```python
from build123d import *

# Parameters (mm, degrees)
SKETCH1_W                = 11
SKETCH1_H                = 10.5
BOSS_EXTRUDE1_DEPTH      = 7.5
SKETCH2_W                = 11
SKETCH2_H                = 10.5
SKETCH2_R                = 2.795278083
CUT_EXTRUDE1_DEPTH       = 6
CUT_EXTRUDE2_DEPTH       = 6
SKETCH5_W                = 5.867744682
SKETCH5_H                = 6.773951876
SKETCH5_W_2              = 3.131118199
SKETCH5_H_2              = 7.595162723
SKETCH5_W_3              = 1.565559099
SKETCH5_H_3              = 1.410160094
SKETCH5_W_4              = 1.497318165
SKETCH5_W_5              = 1.429294678
SKETCH5_W_6              = 1.22939712
BOSS_EXTRUDE2_DEPTH      = 0.5
SKETCH6_R                = 0.720165483
CUT_EXTRUDE3_DEPTH       = 5.5
CUT_EXTRUDE4_START       = -0.5
SKETCH7_W                = 6.315969547
SKETCH7_H                = 7.313839146
SKETCH7_R                = 1.792834501
CUT_EXTRUDE4_DEPTH       = 4.5
SKETCH8_W                = 2.504754688
SKETCH8_H                = 5.654171149
BOSS_EXTRUDE3_DEPTH      = 2.5
CHAMFER1_SIZE            = 0.5
BOSS_EXTRUDE4_DEPTH      = 0.5
BOSS_EXTRUDE4_DEPTH_BACK = 6
SKETCH11_R               = 0.448273795
SKETCH11_R_2             = 0.519161878
SKETCH11_R_3             = 0.470017501
SKETCH11_R_4             = 0.405329815
CUT_EXTRUDE5_DEPTH       = 6
SKETCH12_W               = 15.986280265
SKETCH12_H               = 22.221265256
CUT_EXTRUDE6_DEPTH       = 1
SKETCH14_W               = 2.367247422
SKETCH14_H               = 5.32267157
SKETCH14_W_2             = 2.25297781
SKETCH14_W_3             = 3.874113275
SKETCH14_H_2             = 2.566072862
BOSS_EXTRUDE5_DEPTH      = 1
SKETCH15_W               = 0.295662385
SKETCH15_H               = 1.277257847
SKETCH15_W_2             = 2.29913968
SKETCH15_H_2             = 1.589846546
BOSS_EXTRUDE6_DEPTH      = 0.25


with BuildPart() as part:
    # Sketch1 → Boss-Extrude1 (new body)
    with BuildSketch(Plane(origin=(0, 0, 0), x_dir=(1, 0, 0), z_dir=(0, 1, 0))):
        Rectangle(SKETCH1_W, SKETCH1_H)
    extrude(amount=BOSS_EXTRUDE1_DEPTH)

    # Sketch2 → Cut-Extrude1 (cut)
    with BuildSketch(Plane(origin=(0, 7.5, 0), x_dir=(1, 0, 0), z_dir=(0, 1, 0))):
        Rectangle(SKETCH2_W, SKETCH2_H)
        with Locations(Location((1.820403911, -0.575947, 0), (0, 0, 270))):
            Circle(SKETCH2_R, mode=Mode.SUBTRACT)
    extrude(amount=-CUT_EXTRUDE1_DEPTH, mode=Mode.SUBTRACT)

    # Sketch4 → Cut-Extrude2 (cut)
    with BuildSketch(Plane(origin=(0, 7.5, 0), x_dir=(1, 0, 0), z_dir=(0, 1, 0))):
        with BuildLine():
            Line((3.877357483, 1.31680802), (3.877357483, -2.46870202))
            ThreePointArc((3.877357483, -2.46870202), (4.615681994, -0.575947), (3.877357483, 1.31680802))
        make_face()
        with BuildLine():
            Line((-0.236549661, 1.31680802), (-0.236549661, -2.46870202))
            ThreePointArc((-0.236549661, -2.46870202), (-0.974874172, -0.575947), (-0.236549661, 1.31680802))
        make_face()
    extrude(amount=-CUT_EXTRUDE2_DEPTH, mode=Mode.SUBTRACT)

    # Sketch5 → Boss-Extrude2 (add)
    with BuildSketch(Plane(origin=(0, 1.5, 0), x_dir=(1, 0, 0), z_dir=(0, 1, 0))):
        with Locations((1.820403911, -0.575947)):
            Rectangle(SKETCH5_W, SKETCH5_H)
        with Locations((-3.275534534, -0.986552423)):
            Rectangle(SKETCH5_W_2, SKETCH5_H_2)
        with Locations((-2.492754984, 4.155418326)):
            Rectangle(SKETCH5_W_3, SKETCH5_H_3)
        with Locations((-0.364809348, 4.155418326)):
            Rectangle(SKETCH5_W_4, SKETCH5_H_3)
        with Locations((1.660671656, 4.155418326)):
            Rectangle(SKETCH5_W_5, SKETCH5_H_3)
        with Locations((3.673751281, 4.155418326)):
            Rectangle(SKETCH5_W_6, SKETCH5_H_3)
    extrude(amount=BOSS_EXTRUDE2_DEPTH)

    # Sketch6 → Cut-Extrude3 (cut)
    with BuildSketch(Plane(origin=(0, 7.5, 0), x_dir=(1, 0, 0), z_dir=(0, 1, 0))):
        with Locations((1.820403911, 2.219331083)):
            Circle(SKETCH6_R)
        with Locations((1.820403911, -3.371225083)):
            Circle(SKETCH6_R)
    extrude(amount=-CUT_EXTRUDE3_DEPTH, mode=Mode.SUBTRACT)

    # Sketch7 → Cut-Extrude4 (cut)
    with BuildSketch(Plane(origin=(0, 7.5, 0), x_dir=(1, 0, 0), z_dir=(0, 1, 0)).offset(CUT_EXTRUDE4_START)):
        with Locations((2.565041423, -0.688586972)):
            Rectangle(SKETCH7_W, SKETCH7_H)
        with Locations(Location((1.820403911, -0.575947, 0), (0, 0, 270))):
            Circle(SKETCH7_R, mode=Mode.SUBTRACT)
    extrude(amount=-CUT_EXTRUDE4_DEPTH, mode=Mode.SUBTRACT)

    # Sketch8 → Boss-Extrude3 (add)
    with BuildSketch(Plane(origin=(0, 2, 0), x_dir=(1, 0, 0), z_dir=(0, 1, 0))):
        with Locations((-3.183335966, -1.017589679)):
            Rectangle(SKETCH8_W, SKETCH8_H)
    extrude(amount=BOSS_EXTRUDE3_DEPTH)

    # Chamfer1
    chamfer1_edges = [part.edges().sort_by_distance(p)[0] for p in [
        (-4.43571331, 4.5, 1.017589679),
        (-3.183335966, 4.5, 3.844675254),
        (-1.930958622, 4.5, 1.017589679),
        (-3.183335966, 4.5, -1.809495895),
    ]]
    chamfer(chamfer1_edges, length=CHAMFER1_SIZE)

    # Sketch9 → Boss-Extrude4 (add, two sides: drawn at the far end of the back side and taken through both)
    with BuildSketch(Plane.XY.offset(3.844675254).offset(-BOSS_EXTRUDE4_DEPTH_BACK)):
        with BuildLine():
            Line((-3.65938344, 3.018172096), (-3.960413084, 2))
            Line((-3.960413084, 2), (-2.240880522, 2))
            Line((-2.240880522, 2), (-2.525820591, 3.018172096))
            ThreePointArc((-2.525820591, 3.018172096), (-3.092602015, 3.584953521), (-3.65938344, 3.018172096))
        make_face()
    extrude(amount=BOSS_EXTRUDE4_DEPTH + BOSS_EXTRUDE4_DEPTH_BACK)

    # Sketch11 → Cut-Extrude5 (cut)
    with BuildSketch(Plane(origin=(0, 2, 0), x_dir=(1, 0, 0), z_dir=(0, 1, 0))):
        with Locations(Location((-2.434309819, 4.1008725, 0), (0, 0, 270))):
            Circle(SKETCH11_R)
        with Locations(Location((-0.282142489, 4.1008725, 0), (0, 0, 270))):
            Circle(SKETCH11_R_2)
        with Locations(Location((1.714254577, 4.1008725, 0), (0, 0, 270))):
            Circle(SKETCH11_R_3)
        with Locations(Location((3.740407892, 4.1008725, 0), (0, 0, 270))):
            Circle(SKETCH11_R_4)
    extrude(amount=-CUT_EXTRUDE5_DEPTH, mode=Mode.SUBTRACT)

    # Sketch12 → Cut-Extrude6 (cut)
    with BuildSketch(Plane.XZ):
        with Locations((0.612445896, -2.778297047)):
            Rectangle(SKETCH12_W, SKETCH12_H)
    extrude(amount=-CUT_EXTRUDE6_DEPTH, mode=Mode.SUBTRACT)

    # Sketch14 → Boss-Extrude5 (add)
    with BuildSketch(Plane.XZ.offset(-1)):
        with Locations((-3.713682192, 1.657442308)):
            Rectangle(SKETCH14_W, SKETCH14_H)
        with Locations((-0.626830267, 1.657442308)):
            Rectangle(SKETCH14_W_2, SKETCH14_H)
        with Locations((2.948180384, 1.283036431)):
            Rectangle(SKETCH14_W_3, SKETCH14_H_2)
    extrude(amount=BOSS_EXTRUDE5_DEPTH)

    # Sketch15 → Boss-Extrude6 (add)
    with BuildSketch(Plane.XZ.offset(-1)):
        with Locations((1.762732856, -0.322099443)):
            Rectangle(SKETCH15_W, SKETCH15_H)
        with Locations((2.880831271, -0.322099443)):
            Rectangle(SKETCH15_W, SKETCH15_H)
        with Locations((4.061872536, -0.322099443)):
            Rectangle(SKETCH15_W, SKETCH15_H)
        with Locations((2.912302696, 3.03749296)):
            Rectangle(SKETCH15_W_2, SKETCH15_H_2)
    extrude(amount=BOSS_EXTRUDE6_DEPTH)


solid = part.part
```
Design review of the part built by this model. Coordinates are the model's own, in mm. A direction names the side the tool comes from. Round coordinates to 2 decimals unless told otherwise and drop trailing zeros. Write each loop counter-clockwise with the first axis right and the second up, starting at its lowest first coordinate (ties: lowest second). Pieces come first, ordered by that corner, then holes.
Item 1: We need section A-A on y = 2.25. Write out the cut boundary in (x, z), and give its area (3 significant figures).
Item 2: We need section C-C on y = 1.25. Write out the cut boundary in (x, z), and give its area (3 significant figures).
Item 3: The part is to be moulded in two halves that separate along X. For faces 1 (the cylindrical face through (-0.126, 1.507, -3.606)), 2 (the flat face through (-4.897, 0.5, 1.6)), 3 (the flat face through (4.885, 0.5, 1.3)), 4 (the flat face through (3, 0, 1)), say which applies: +X half, -X half, draft (parallel to the pull), parting line (faces both ways), or undercut.
Item 4: For probe 1 along Y at (x, z) = (1, -1.25); probe 2 along Y at (x, z) = (-4, 4); probe 3 along Z at (x, y) = (-1.25, 0.75), list the stretches that pass through material, from the lowest coordinate up.
Item 5: For faces 5 (the flat face through (-3, 4.5, 1)), 6 (the cylindrical face through (0.07, 4.78, 0.19)), 7 (the cylindrical face through (0.386, 7.254, -1.823)), 8 (the cylindrical face through (3.25, 7.25, 2.98)), 9 (the cylindrical face through (3.273, 2.254, -1.812)), list the 3-axis set-ups (+Z, -Z, +X, -X, +Y, -Y) from which the entire face can be reached by the end or side of a thin tool; tool diameter is ignored.
Item 6: We need section D-D on x = -3.5. Write out the cut boundary in (y, z), and give its area (3 significant figures).
Item 7: Clearance check with flat-ended pins moving along their axes: pin 1 Ø1.6 at (x, y) = (-3, 3) entering from -Z; pin 2 Ø5 at (x, z) = (-4.5, 3) entering from +Y; pin 3 Ø3 at (x, z) = (2.5, -2) entering from -Y. State where each tip first meets the part, or that it passes through.
Returned:
1. outline: (-4.44, -1.81) - (-3.89, -1.81) - (-3.89, -2.16) - (-2.31, -2.16) - (-2.31, -1.81) - (-1.93, -1.81) - (-1.93, 3.84) - (-2.31, 3.84) - (-2.31, 4.34) - (-3.89, 4.34) - (-3.89, 3.84) - (-4.44, 3.84) - close; (-0.24, -1.32) arc R2.8 ccw to (1.11, -2.13) arc R0.72 cw to (2.53, -2.13) arc R2.8 ccw to (3.88, -1.32) - (3.88, 2.47) arc R2.8 ccw to (2.53, 3.28) arc R0.72 cw to (1.11, 3.28) arc R2.8 ccw to (-0.24, 2.47) - close
1. area: 34.7 mm2
2. outline: (-5.5, -5.25) - (5.5, -5.25) - (5.5, 5.25) - (-5.5, 5.25) - close; hole circle Ø0.9 at (-2.43, -4.1); hole circle Ø1.04 at (-0.28, -4.1); hole circle Ø0.94 at (1.71, -4.1); hole circle Ø0.81 at (3.74, -4.1)
2. area: 113 mm2
3. face 1: undercut
3. face 2: -X half
3. face 3: +X half
3. face 4: draft
4. probe 1: y = 1 to 2.5, 7 to 7.5
4. probe 2: y = 0 to 2
4. probe 3: z = -1 to 4.32
5. face 5: +Z, -Z, -X, +Y
5. face 6: none
5. face 7: -Z, -X, +Y
5. face 8: +Z, +X, +Y
5. face 9: -Z, +X, +Y
6. outline: (0, -1) - (1, -1) - (1, -5.25) - (1.5, -5.25) - (1.5, -2.81) - (2, -2.81) - (2, -2.16) - (3.41, -2.16) - (3.41, -1.81) - (4, -1.81) - (4.5, -1.31) - (4.5, 3.34) - (4, 3.84) - (3.41, 3.84) - (3.41, 4.34) - (2, 4.34) - (2, 4.78) - (1.5, 4.78) - (1.5, 5.25) - (1, 5.25) - (1, 4.32) - (0, 4.32) - close
6. area: 29.5 mm2
7. pin 1: stops at z = -2.16
7. pin 2: stops at y = 4.5
7. pin 3: stops at y = 0.75
